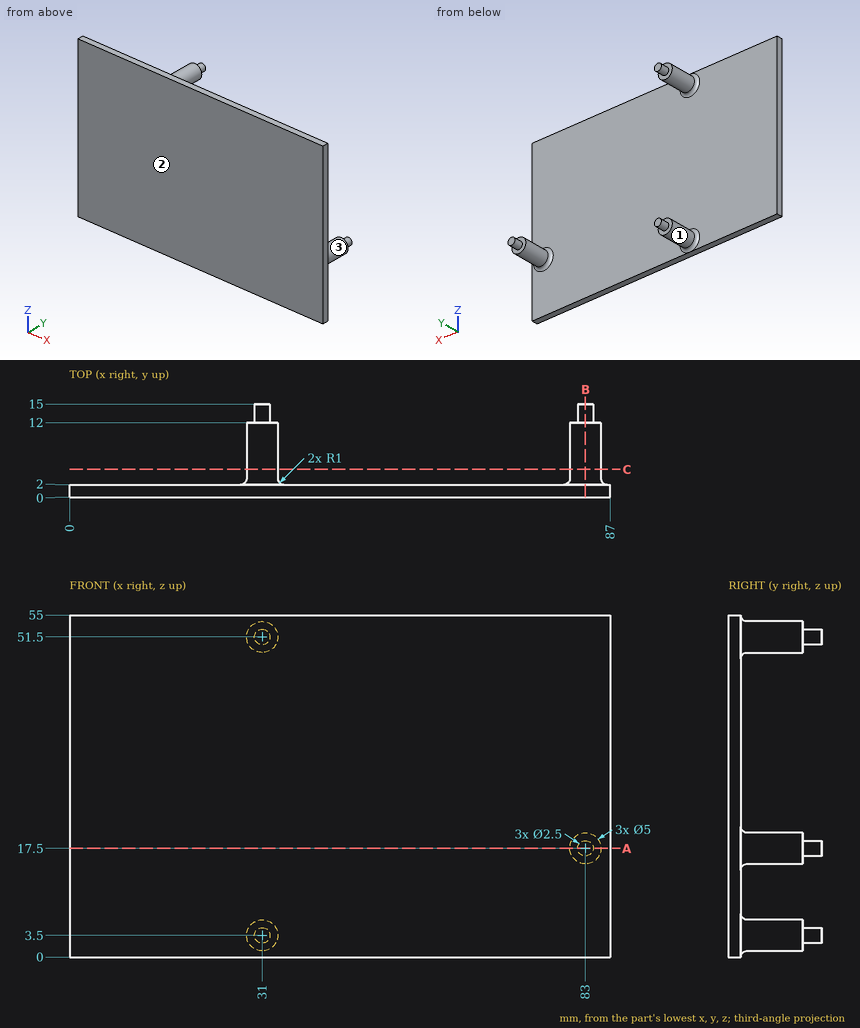
Can you work these out from the drawing? Everything is in mm from the part's minimum corner. Coordinates: 2 decimals unless noted, no trailing zeros. Loops run counter-clockwise (first coordinate to the right, second up) from the corner with the lowest first, then second, coordinate; pieces in that order, holes last. Notation, with made-up numbers: M 25,-33 L 82,-33 A14 cw 82,-11 Z; hole C 78.5,83.25 d10. An arc over 180 degrees is marked long. Put each result on its own line as item: value. Start each with the question number.
(1) Thinking about a two-plate mould opening in Z: for the marked faces 1, 2 and 3, which applies, pulls with the +Z half, pulls with the -Z half, needs draft (parallel to the pull), parting line crosses it, or undercut?
(2) Suppose I cut it at B-B on x = 83. Please give me the cut outline in (y, z), then the cut area to 3 significant figures.
(3) Suppose I cut it at A-A on z = 17.5. Please give me the cut outline in (x, y), then the cut area to 3 significant figures.
(4) I need wall thicknesses on line 1 (Y direction, x = 21.5, z = 6.5). Which ranges of the line are inside material? Lowest first, please. Write a range as from..to.
(5) Will this pin go through, and if not, where does the flat tip stop? P1, Ø16.5, axis at x = 63, z = 15, coming from the +Y side.
(6) Suppose I cut it at C-C on y = 4.5. Please give me the cut outline in (x, z).
Solutions:
1. face 1: undercut
1. face 2: needs draft
1. face 3: parting line crosses it
2. outline: M 0,0 L 2,0 L 2,14 A1 cw 3,15 L 12,15 L 12,16.25 L 15,16.25 L 15,18.75 L 12,18.75 L 12,20 L 3,20 A1 cw 2,21 L 2,55 L 0,55 Z
2. area: 168 mm2
3. outline: M 0,0 L 87,0 L 87,2 L 86.5,2 A1 cw 85.5,3 L 85.5,12 L 84.25,12 L 84.25,15 L 81.75,15 L 81.75,12 L 80.5,12 L 80.5,3 A1 cw 79.5,2 L 0,2 Z
3. area: 232 mm2
4. line 1: y = 0..2
5. P1: stops at y = 2
6. outline: C 31,3.5 d5; C 31,51.5 d5; C 83,17.5 d5
